For this review, take the finished solid that the model builds, in its own axes (mm). Face numbers are marked on the shaded views. A direction names the side the tool comes from. Round coordinates to 2 decimals unless told otherwise and drop trailing zeros. Order: outer loops, then holes, each group sorted by start corner. A loop starts at its lowest first (then second) coordinate and runs counter-clockwise, first axis right, second up.
```python
from build123d import *

# Parameters (mm, degrees)
F0_R        = 3.75
F1_DEPTH    = 2
F2_R        = 1.9
F3_DEPTH    = 14
F4_S5_R     = 1.9
F4_T6_DEPTH = 7


# Not quite as in the source:
# - a fillet or chamfer that OpenCascade refuses, or shapes differently, is made with other operations: its cross-section is extruded or revolved along the edge and cut away or added


with BuildPart() as f1:
    # F0 (on Top) → F1 (new body)
    with BuildSketch(Plane.XY):
        Circle(F0_R)
    extrude(amount=F1_DEPTH)

    # F2 (on face) → F3 (join)
    with BuildSketch(Plane(origin=(0, 0, 0), x_dir=(1, 0, 0), z_dir=(0, 0, -1))):
        Circle(F2_R)
    extrude(amount=F3_DEPTH)

    # F4: chamfer of 2 on 1 edges, made by hand


with BuildPart() as f4_tool2:
    # F4_s3 → F4_t4 (revolve)
    with BuildSketch(Plane.XZ):
        Polygon((3.75, 2), (1.75, 0), (3.75, 0), align=None)
    revolve(axis=Axis((0, 0, 0), (0, 0, 1)))

    # F4_s5 → F4_t6 (cut, symmetric)
    with BuildSketch(Plane.XY.offset(1)):
        Circle(F4_S5_R)
    extrude(amount=F4_T6_DEPTH, both=True, mode=Mode.SUBTRACT)


with BuildPart() as f1_1:
    add(f1.part)

    # F4_t1: cut F4_tool2
    add(f4_tool2.part, mode=Mode.SUBTRACT)


solid = f1_1.part
```
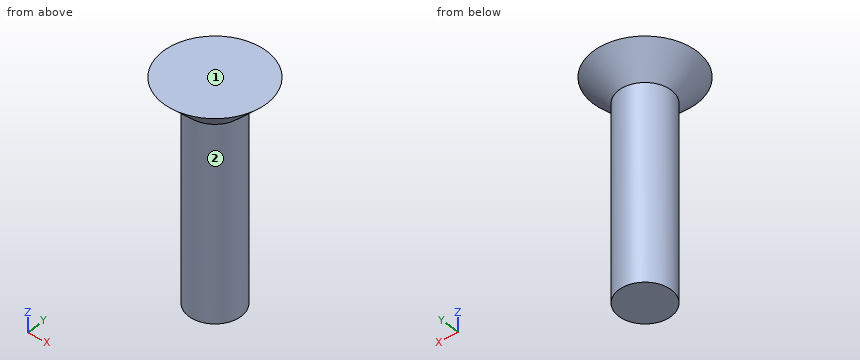
Q1. Tool access review of the marked faces 1 and 2: name each direction out of +Z, -Z, +X, -X, +Y, -Y from which nothing blocks a thin tool from reaching the whole face with its end or side.
Q2. Take a section at A-A, the plane x = 0. State the section outline as (y, z) points.
Q3. Take a section at D-D, the plane z = 0.5. State the section outline as (x, y) points.
Q4. Take a section at C-C, the plane z = -3.75. State the section outline as (x, y) points, plus the area to 3 significant figures.
Q5. Wall thickness on line 1 (X direction, y = 0, z = -8.25); line 2 (Z direction, x = 1.5, y = 2.75); line 3 (X direction, y = -1.5, z = 0.25): over which ranges is each line inside the solid? List them lowest first.
Q6. Clearance check with flat-ended pins moving along their axes: pin 1 (2 mm diameter, centred on x = 2, z = -10.5, fed in from +Y); pin 2 (3 mm diameter, centred on y = 2.5, z = -4.5, fed in from +X); pin 3 (4 mm diameter, centred on y = 0.5, z = -5.5, fed in from +X). State where each tip first meets the part, or that it passes through.
Working result:
1. face 1: +Z, +X, -X, +Y, -Y
1. face 2: -Z
2. outline: (-3.75, 2) - (-1.9, 0.15) - (-1.9, -14) - (1.9, -14) - (1.9, 0.15) - (3.75, 2) - close
3. outline: circle Ø4.5 at (0, 0)
4. outline: circle Ø3.8 at (0, 0)
4. area: 11.3 mm2
5. line 1: x = -1.9 to 1.9
5. line 2: z = 1.38 to 2
5. line 3: x = -1.32 to 1.32
6. pin 1: stops at y = 1.62
6. pin 2: stops at x = 1.62
6. pin 3: stops at x = 1.9
